CAD build for the part. Positions are in the model's coordinates, mm. A direction names the side the tool comes from. Give positions to 0.01 mm unless a question says otherwise; leave off trailing zeros. Order: outer loops, then holes, each group sorted by start corner. A loop starts at its lowest first (then second) coordinate and runs counter-clockwise, first axis right, second up.
Item 1: Band-saw the part on C-C on z = -16. Give the cut face in (x, y).
Item 2: Which spindle directions (+Z, -Z, +X, -X, +Y, -Y) get a long thin tool onto all of the face, cutting with end or side? Do faces 1 (the flat face through (-26.929, 62.611, -18.794)), 2 (the flat face through (-66, 63, -10.838)), 3 (the flat face through (0, 63, -28.702)). Say none if no direction does.
Item 3: Wall check: L1, parallel to X at y = 101, z = -24.5; L2, parallel to Z at x = -74, y = 8.5; L3, parallel to X at y = 70.5, z = -22.5. Give the ranges that are in metal, low to high.
Item 4: Band-saw the part on B-B on x = 8.5. Give the cut face in (y, z), plus the area to 3 significant figures.
Item 5: Two-plate mould, pull along Z, no slides. Class faces 4 (the flat face through (6, 63, -4.762)), 5 (the flat face through (-24, 0, -21.3)), 6 (the flat face through (-65, 63, -8.128)), 7 (the flat face through (14.668, 63, -17)): released by +Z, released by -Z, zero draft, split by the parting line, or undercut.
Item 6: Flat gauge pins, fed straight in: P1, Ø2, axis at x = -23, y = 29, coming from the -Z side; P2, Ø1.5, axis at x = -33, y = 53, coming from the +Z side; P3, Ø4.5, axis at x = 9, y = 86, coming from the +Z side. Where does each tip first touch, or does it go through?
Item 7: Band-saw the part on D-D on x = -10.5. Give the cut face in (y, z).
```python
from build123d import *

# Parameters (mm, degrees)
F0_R     = 3.175
F1_DEPTH = 127
F2_R     = 3.9624
F3_R     = 1.524


# Not quite as in the source:
# - a feature names something its author has since deleted; it is built from what else it names


with BuildPart() as f1:
    # F0 (on Front) → F1 (new body)
    with BuildSketch(Plane.XZ):
        with BuildLine():
            ThreePointArc((4.7011447808, -0.762), (4.7471364141, -0.3822330647), (4.7625, 0))
            ThreePointArc((4.7625, 0), (-3.3675960454, 3.3675960454), (0, -4.7625))
            ThreePointArc((0, -4.7625), (3.0864527576, -3.6270119417), (4.7011447808, -0.762))
        make_face()
        Circle(F0_R, mode=Mode.SUBTRACT)
        with BuildLine():
            ThreePointArc((4.7011447808, -0.762), (3.0864527576, -3.6270119417), (0, -4.7625))
            Line((0, -4.7625), (14.6685, -4.7625))
            Line((14.6685, -4.7625), (14.6685, -28.702))
            Line((14.6685, -28.702), (-13.6858972215, -28.702))
            Line((-13.6858972215, -28.702), (-41.1854304771, -8.128))
            Line((-41.1854304771, -8.128), (-88.58598171, -8.128))
            Line((-88.58598171, -8.128), (-88.58598171, -10.83818))
            Line((-88.58598171, -10.83818), (-42.8310789114, -10.83818))
            Line((-42.8310789114, -10.83818), (-15.3315456557, -31.41218))
            Line((-15.3315456557, -31.41218), (17.4625, -31.41218))
            Line((17.4625, -31.41218), (17.4625, -0.762))
            Line((17.4625, -0.762), (4.7011447808, -0.762))
        make_face()
    extrude(amount=-F1_DEPTH)

    # F2
    f2_edges = [f1.edges().sort_by_distance(p)[0] for p in [
        (17.4625, 63.5, -0.762),
        (-15.331546, 63.5, -31.41218),
        (-41.18543, 63.5, -8.128),
        (17.4625, 63.5, -31.41218),
    ]]
    fillet(f2_edges, radius=F2_R)

    # F3
    f3_edges = [f1.edges().sort_by_distance(p)[0] for p in [
        (14.6685, 63.5, -4.7625),
        (-13.685897, 63.5, -28.702),
        (-42.831079, 63.5, -10.83818),
        (14.6685, 63.5, -28.702),
    ]]
    fillet(f3_edges, radius=F3_R)


solid = f1.part
```
The answers:
1. outline: (-35.93, 0) - (-30.66, 0) - (-30.66, 127) - (-35.93, 127) - close; (14.67, 0) - (17.46, 0) - (17.46, 127) - (14.67, 127) - close
2. face 1: +Z, +Y, -Y
2. face 2: -Z, -X, +Y, -Y
2. face 3: +Y, -Y
3. L1: x = -24.57 to -19.3, 14.67 to 17.46
3. L2: z = -10.84 to -8.13
3. L3: x = -27.24 to -21.98, 14.67 to 17.46
4. outline: (0, -31.41) - (127, -31.41) - (127, -28.7) - (0, -28.7) - close; (0, -4.76) - (127, -4.76) - (127, -0.76) - (0, -0.76) - close
4. area: 852 mm2
5. face 4: undercut
5. face 5: zero draft
5. face 6: released by +Z
5. face 7: undercut
6. P1: stops at z = -26.42
6. P2: stops at z = -13.69
6. P3: stops at z = -0.76
7. outline: (0, -31.41) - (127, -31.41) - (127, -28.7) - (0, -28.7) - close
